Autodesk Inventor part; units mm, degrees
ref_plane "YZ Plane" through (0, 0, 0) normal (1, 0, 0) x (0, 1, 0)
ref_plane "XZ Plane" through (0, 0, 0) normal (0, 1, 0) x (-1, 0, 0)
ref_plane "XY Plane" through (0, 0, 0) normal (0, 0, 1) x (1, 0, 0)
sketch "Sketch1" plane through (0, 0, 0) normal (0, 0, 1) x (1, 0, 0)
  line L0 (0, 0) -> (15, 0)
  line L1 (15, 0) -> (15, 4)
  line L2 (15, 4) -> (0, 4)
  line L3 (0, 4) -> (0, 0)
  line L4 (0, 53.5) -> (15, 53.5)
  line L5 (15, 53.5) -> (15, 49.5)
  line L6 (15, 49.5) -> (0, 49.5)
  line L7 (0, 49.5) -> (0, 53.5)
  line L8 (0, 53.5) -> (-4.3, 53.5)
  line L9 (-4.3, 53.5) -> (-4.3, -6.5)
  line L10 (-4.3, -6.5) -> (0, -6.5)
  line L11 (0, -6.5) -> (0, 53.5)
  point P0 (0, 49.5)
  dimension "d0" = 15
  dimension "d1" = 4
  dimension "d2" = 15
  dimension "d3" = 4
  dimension "d4" = 45.5
  dimension "d5" = 4.3
  dimension "d6" = 60
extrude "Extrusion1" add sketch "Sketch1" along normal mid plane 45
extrude "Extrusion2" cut sketch "Sketch1" along normal mid plane 30 contours L3 L2 L1 L0
sketch "Sketch3" plane through (0, 49.5, 22.5) normal (0, -1, 0) x (1, 0, 0)
  line L0 (0, 0) -> (15, 0)
  line L1 (7.5, 0) -> (7.5, -45)
  line L2 (15, -45) -> (0, -45)
  circle A0 centre (7.5, -3.75) radius 1.55
  circle A1 centre (7.5, -7.5) radius 1.55
  circle A2 centre (7.5, -22.5) radius 1.55
  circle A3 centre (7.5, -37.5) radius 1.55
  circle A4 centre (7.5, -41.25) radius 1.55
  line L3 (0, 0) -> (15, 0)
  line L4 (15, -45) -> (0, -45)
  line L5 (15, -45) -> (15, 0)
  point P0 (0, -22.5)
  dimension "d11" = 3.1
  dimension "d12" = 3.1
  dimension "d13" = 3.1
  dimension "d14" = 3.1
  dimension "d15" = 3.1
  dimension "d16" = 3.75
  dimension "d17" = 7.5
  dimension "d18" = 3.75
  dimension "d19" = 7.5
  dimension "d20" = 7.5
extrude "Extrusion3" cut sketch "Sketch3" along normal through all contours A0 L1 | L1 A0 | A4 L1 | L1 A4
extrude "Extrusion4" cut sketch "Sketch3" against normal through all contours A1 L1 | L1 A1 | A2 L1 | L1 A2 | A3 L1 | L1 A3
sketch "Sketch4" plane through (0, 4, -22.5) normal (1, 0, 0) x (0, 0, -1)
  circle A0 centre (-22.5, 1.25) radius 6
  line L0 (-45, -10.5) -> (0, -10.5)
  line L1 (-22.5, 1.25) -> (-22.5, -10.5) construction
  point P0 (-22.5, -4)
  dimension "d29" = 12
  dimension "d40" = 11.75
extrude "Extrusion6" cut sketch "Sketch4" against normal through all
fillet "Fillet1" radius 2 14 edges at (0, 49.5, 0) (15, 49.5, 0) (15, 53.5, 0) (-4.3, 53.5, 0) (0, 4, 18.75) (0, 4, -18.75) (15, 4, -18.75) (15, 0, -18.75) (15, 4, 18.75) (15, 0, 18.75) (0, -6.5, 0) (0, 0, 18.75) (0, 0, -18.75) (-4.3, -6.5, 0)
properties part number "BearingBracket" material "PC/ABS Plastic"
Build history of the part. All positions in model axes, mm. A direction names the side the tool comes from. Give positions to 0.01 mm unless a question says otherwise; leave off trailing zeros. Loops run counter-clockwise (first coordinate to the right, second up) from the corner with the lowest first, then second, coordinate; pieces in that order, holes last.
1) Band-saw the part on A-A on y = 5.25. List the corners of the cut face in (x, z).
Values follow:
outline: (-4.3, -22.5) - (0.15, -22.5) - (0.15, -15) - (0, -15) - (0, -6) - (-4.3, -6) - close; (-4.3, 6) - (0, 6) - (0, 15) - (0.15, 15) - (0.15, 22.5) - (-4.3, 22.5) - close
2) 3-axis set-ups, long thin cutter, end or side, ignore diameter. For faces 1 (the face through (7.298, 2.028, -20.287)), 2 (the face through (8.978, 51.472, 0.466)), 3 (the face through (6, 0, -20)), 4 (the face through (14.4, 3.43, 18.7)): which of +Z, -Z, +X, -X, +Y, -Y reach the whole face in a straight line?
Values follow:
face 1: -Y
face 2: +Y, -Y
face 3: +Z, -Z, +X, -Y
face 4: +Z, -Z, +X
3) Band-saw the part on C-C on x = 7. State how many separate pieces and enclosed holes the cut face has, then the cut area to 3 significant figures.
Values follow:
separate pieces: 8
enclosed holes: 0
area: 181 mm2
4) Two-plate mould, pull along X, no slides. Class faces 5 (the face through (7.298, 51.472, 16.537)), 6 (the face through (-2.12, 9.31, 4.42)), 7 (the face through (7.298, 51.472, -13.463)), 8 (the face through (0.57, -0.6, -18.8)): released by +X, released by -X, zero draft, split by the parting line, or undercut.
Values follow:
face 5: undercut
face 6: zero draft
face 7: undercut
face 8: released by +X
5) Drop flat-ended pins along their axis: P1, Ø1.9, axis at x = 7.5, z = -15, coming from the +Y side; P2, Ø3, axis at y = 36, z = -3.5, coming from the +X side; P3, Ø5.5, axis at x = 8, z = -10, coming from the -Y side. Give the stop position or say it passes through.
Values follow:
P1: stops at y = 4
P2: stops at x = 0
P3: stops at y = 49.5
6) Probe line 1 along Z through (x, y) = (7.5, 52.3); line 2 along Z through (x, y) = (7.5, 2.7); line 3 along X through (y, z) = (1.9, 18.75). List the from-to ranges inside material, lowest first.
Values follow:
line 1: z = -22.5 to -16.55, -13.45 to -1.55, 1.55 to 13.45, 16.55 to 22.5
line 2: z = -22.5 to -20.3, -17.2 to -15, 15 to 17.2, 20.3 to 22.5
line 3: x = -4.3 to 5.95, 9.05 to 15
